```python
from build123d import *

# Parameters (mm, degrees)
SKETCH_1_R      = 1.5
EXTRUDE_1_DEPTH = 3


with BuildPart() as part:
    # 草图1 → 凸台-拉伸1 (new body)
    with BuildSketch(Plane(origin=(0, 0, 0), x_dir=(1, 0, 0), z_dir=(0, 1, 0))):
        with BuildLine():
            Line((10, 0), (136.884360712, 0))
            ThreePointArc((136.884360712, 0), (137.900113715, -0.277140216), (138.634360712, -1.031754163))
            Line((138.634360712, -1.031754163), (139.429147615, -2.468245837))
            ThreePointArc((139.429147615, -2.468245837), (140.163394612, -3.222859784), (141.179147615, -3.5))
            Line((141.179147615, -3.5), (168.820852385, -3.5))
            ThreePointArc((168.820852385, -3.5), (169.836605388, -3.222859784), (170.570852385, -2.468245837))
            Line((170.570852385, -2.468245837), (171.365639288, -1.031754163))
            ThreePointArc((171.365639288, -1.031754163), (172.099886285, -0.277140216), (173.115639288, 0))
            Line((173.115639288, 0), (300, 0))
            ThreePointArc((300, 0), (307.071067812, -2.928932188), (310, -10))
            Line((310, -10), (310, -210))
            ThreePointArc((310, -210), (307.071067812, -217.071067812), (300, -220))
            Line((300, -220), (10, -220))
            ThreePointArc((10, -220), (2.928932188, -217.071067812), (0, -210))
            Line((0, -210), (0, -10))
            ThreePointArc((0, -10), (2.928932188, -2.928932188), (10, 0))
        make_face()
        with Locations(Location((14, -14, 0), (0, 0, 270))):
            Circle(SKETCH_1_R, mode=Mode.SUBTRACT)
        with Locations(Location((14, -206, 0), (0, 0, 270))):
            Circle(SKETCH_1_R, mode=Mode.SUBTRACT)
        with Locations(Location((296, -206, 0), (0, 0, 270))):
            Circle(SKETCH_1_R, mode=Mode.SUBTRACT)
        with Locations(Location((296, -12.28568254, 0), (0, 0, 270))):
            Circle(SKETCH_1_R, mode=Mode.SUBTRACT)
        with Locations(Location((155, -206, 0), (0, 0, 270))):
            Circle(SKETCH_1_R, mode=Mode.SUBTRACT)
        with Locations(Location((175, -14, 0), (0, 0, 270))):
            Circle(SKETCH_1_R, mode=Mode.SUBTRACT)
        with Locations(Location((135, -14, 0), (0, 0, 270))):
            Circle(SKETCH_1_R, mode=Mode.SUBTRACT)
        with Locations(Location((296, -110, 0), (0, 0, 270))):
            Circle(SKETCH_1_R, mode=Mode.SUBTRACT)
        with Locations(Location((14, -110, 0), (0, 0, 270))):
            Circle(SKETCH_1_R, mode=Mode.SUBTRACT)
        Polygon((184.455213096, -18.25), (188.75, -14.75), (285, -14.75), (285, -195), (25, -195), (25, -14.75), (119.25, -14.75), (123.544786904, -18.25), (141.179147615, -18.25), (168.820852385, -18.25), align=None, mode=Mode.SUBTRACT)
    extrude(amount=EXTRUDE_1_DEPTH)


solid = part.part
```
Verification items for the finished model (mm, model axes). Give positions to 0.01 mm unless a question says otherwise; leave off trailing zeros. Order: outer loops, then holes, each group sorted by start corner. A loop starts at its lowest first (then second) coordinate and runs counter-clockwise, first axis right, second up. Notation, with made-up numbers: (55.5, 50) -> (113.5, 50) arc R14 ccw to (113.5, 72) -> close; hole circle Ø4 at (85.25, 46.5). An arc over 180 degrees is marked (long way). Use a Markdown table: item, result.
1) Section check A-A, the plane x = 196.5. Record the boundary of the cut face in (y, z), then the cut area to 3 significant figures.
Results:
| item | result |
|---|---|
| outline | (0, 0) -> (3, 0) -> (3, 14.75) -> (0, 14.75) -> close; (0, 195) -> (3, 195) -> (3, 220) -> (0, 220) -> close |
| area | 119 mm² |
2) Depth check by flat-ended pin: pin 1 Ø2.5 at (x, z) = (14, 110) entering from -Y. Enter the tip coordinate at first touch or a pass-through.
Results:
| item | result |
|---|---|
| pin 1 | through |
3) Section check B-B, the plane z = 170. Record the boundary of the cut face in (x, y), then the cut area to 3 significant figures.
Results:
| item | result |
|---|---|
| outline | (0, 0) -> (25, 0) -> (25, 3) -> (0, 3) -> close; (285, 0) -> (310, 0) -> (310, 3) -> (285, 3) -> close |
| area | 150 mm² |
4) Section check C-C, the plane y = 1.6. Give the number of separate pieces and of enclosed holes in the cut face, then the cut area to 3 significant figures.
Results:
| item | result |
|---|---|
| separate pieces | 1 |
| enclosed holes | 10 |
| area | 21,300 mm² |
5) Material ranges on probe 1 along Z at (x, y) = (135, 0.75); probe 2 along X at (y, z) = (1.8, 206); probe 3 along X at (y, z) = (1.3, 110), recorded low to high.
Results:
| item | result |
|---|---|
| probe 1 | 0 to 12.5, 15.5 to 18.25, 195 to 220 |
| probe 2 | 0 to 12.5, 15.5 to 153.5, 156.5 to 294.5, 297.5 to 310 |
| probe 3 | 0 to 12.5, 15.5 to 25, 285 to 294.5, 297.5 to 310 |
